Autodesk Inventor part; units mm, degrees
ref_plane "YZ Plane" through (0, 0, 0) normal (1, 0, 0) x (0, 1, 0)
ref_plane "XZ Plane" through (0, 0, 0) normal (0, 1, 0) x (-1, 0, 0)
ref_plane "XY Plane" through (0, 0, 0) normal (0, 0, 1) x (1, 0, 0)
sketch "スケッチ2" plane through (0, 0, 0) normal (0, 1, 0) x (-1, 0, 0)
  circle A0 centre (0, 0) radius 86.2565
  circle A1 centre (0, 0) radius 70
  circle A2 centre (0, 0) radius 57.5
  line L0 (0, 0) -> (0, 86.2565)
  line L1 (-14.9, 55.5359) -> (-14.9, 84.9598)
  line L2 (14.9, 55.5359) -> (14.9, 84.9598)
  line L3 (14.9, 84.9598) -> (-14.9, 84.9598)
  line L4 (-14.9, 84.9598) -> (-14.9, 115)
  line L5 (-14.9, 115) -> (14.9, 115)
  line L6 (14.9, 115) -> (14.9, 84.9598)
  line L7 (0, 115) -> (7.525, 115)
  line L8 (7.525, 115) -> (7.525, 91.2565)
  line L9 (7.525, 91.2565) -> (0, 91.2565)
  line L10 (0, 91.2565) -> (0, 115)
  line L11 (-7.525, 115) -> (-7.525, 91.2565)
  line L12 (-7.525, 91.2565) -> (0, 91.2565)
  dimension "d8" = 115
  dimension "d6" = 172.513
  dimension "d7" = 140
  dimension "d9" = 14.9
  dimension "d11" = 7.525
  dimension "d12" = 5
  dimension "d13" = 115
extrude "押し出し2" add sketch "スケッチ2" along normal blind 59.1 contours L3 L0 A0 | L2 A1 L0 L3 | A0 L4 L5 L11 L12 L9 L8 L6 | L3 L0 A1 L1 | A0 L0 L3 | L2 A2 L0 A1 | A1 L0 A2 L1
sketch "スケッチ3" plane through (0, 59.1, 0) normal (0, 1, 0) x (1, 0, 0)
  circle A0 centre (0, 0) radius 70
  arc A1 (-14.9, -55.5359) -> (14.9, -55.5359) centre (0, 0) ccw
  circle A2 centre (0, 0) radius 57.5
  line L0 (-14.9, -55.5359) -> (-14.9, -68.3958)
  line L1 (14.9, -55.5359) -> (14.9, -68.3958)
  dimension "d16" = 140
extrude "押し出し3" cut sketch "スケッチ3" against normal blind 9.2 contours L0 A1 L1 A0
fillet "フィレット1" radius 2 8 edges at (-7.525, 29.55, 115) (7.525, 29.55, 115) (14.9, 29.55, 115) (-14.9, 29.55, 115) (14.9, 54.5, 68.3958) (-14.9, 54.5, 68.3958) (14.9, 24.95, 55.5359) (-14.9, 24.95, 55.5359)
properties part number "zigu2"
Read the model definition and answer for the solid it produces. Units are mm, in the model's axes. A direction names the side the tool comes from. Coordinates: 2 decimals unless noted, no trailing zeros. Write each loop counter-clockwise with the first axis right and the second up, starting at its lowest first coordinate (ties: lowest second). Pieces come first, ordered by that corner, then holes. Notation, with made-up numbers: M -18,5 L 34,5 A32 cw 34,37 Z; hole C 19,57 d5. An arc over 180 degrees is marked long. Use a Markdown table: item, result.
Q1. The part is cut by section C-C, the plane z = 66.5. Write down the section's boundary in (x, y), then the cut area to 3 significant figures.
Answer block:
| item | result |
|---|---|
| outline | M -14.9,0 L 14.9,0 L 14.9,49.9 L -14.9,49.9 Z |
| area | 1,490 mm2 |
Q2. Straight lines are drawn through the part: L1, parallel to X at y = 27, z = 95 (3 decimals); L2, parallel to Y at x = -13.5, z = 67; L3, parallel to Z at x = -13, y = 24. For each, find the intervals that lie inside material, in ascending order. Write a range as [from, to].
Answer block:
| item | result |
|---|---|
| L1 | x = [-14.9, -7.525], [7.525, 14.9] |
| L2 | y = [0, 49.9] |
| L3 | z = [56.09, 115] |
Q3. Determine the mould class of faces 1 (the face through (-14.33, 29.96, 114.4)), 2 (the face through (-11, 29, 115)), 3 (the face through (14.9, 29, 85)), 4 (the face through (0, 29, 91.256)) for opening direction X: released by +X, released by -X, zero draft, split by the parting line, or undercut.
Answer block:
| item | result |
|---|---|
| face 1 | released by -X |
| face 2 | zero draft |
| face 3 | released by +X |
| face 4 | undercut |
Q4. The part is cut by section B-B, the plane y = 24. Write down the section's boundary in (x, z) (1 decimal), then the cut area to 3 significant figures.
Answer block:
| item | result |
|---|---|
| outline | M -14.9,58.1 A2 ccw -12.5,56.1 A57.5 cw 12.5,56.1 A2 ccw 14.9,58.1 L 14.9,113 A2 ccw 12.9,115 L 9.5,115 A2 ccw 7.5,113 L 7.5,91.3 L -7.5,91.3 L -7.5,113 A2 ccw -9.5,115 L -12.9,115 A2 ccw -14.9,113 Z |
| area | 1,370 mm2 |
Q5. Each of these flat-tipped pins is pushed along its axis until it touches: pin 1 Ø10 at (x, z) = (5.5, 94.5) entering from -Y; pin 2 Ø5 at (x, y) = (2.5, 49.5) entering from -Z; pin 3 Ø4.5 at (x, y) = (0, 17.5) entering from +Z. Where does it stop, or does it pass through?
Answer block:
| item | result |
|---|---|
| pin 1 | stops at y = 0 |
| pin 2 | stops at z = 57.28 |
| pin 3 | stops at z = 91.26 |
Q6. The part is cut by section A-A, the plane z = 94.5. Write down the section's boundary in (x, y) (3 decimals), then the cut area to 3 significant figures.
Answer block:
| item | result |
|---|---|
| outline | M -14.9,0 L -7.525,0 L -7.525,59.1 L -14.9,59.1 Z; M 7.525,0 L 14.9,0 L 14.9,59.1 L 7.525,59.1 Z |
| area | 872 mm2 |
Q7. The part is cut by section D-D, the plane x = -6.5. Write down the section's boundary in (y, z), then the cut area to 3 significant figures.
Answer block:
| item | result |
|---|---|
| outline | M 0,57.13 L 49.9,57.13 L 49.9,69.7 L 59.1,69.7 L 59.1,91.26 L 0,91.26 Z |
| area | 1,900 mm2 |
Q8. Which of the six approach directions +Z, -Z, +X, -X, +Y, -Y give full straight-line access (tool end or side, diameter ignored) to faces 5 (the face through (14.3, 29.96, 114.43)), 6 (the face through (-8.126, 29.964, 114.43))?
Answer block:
| item | result |
|---|---|
| face 5 | +Z, +X, +Y, -Y |
| face 6 | +Z, +Y, -Y |
